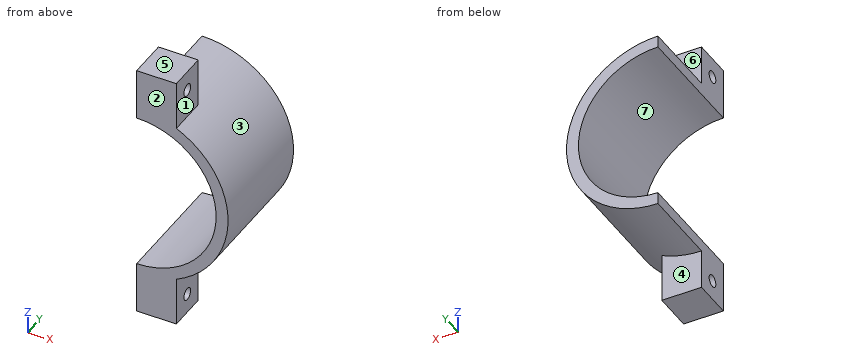
```python
from build123d import *

# Parameters (mm, degrees)
TUBE_DEPTH         = 30
TERMINALS_DEPTH    = 10
CUT_EXTRUDE1_REACH = 25
SKETCH3_R          = 1.524


with BuildPart() as part:
    # Sketch1 → Tube (new body)
    with BuildSketch(Plane(origin=(0, 0, 0), x_dir=(1, 0, 0), z_dir=(0, 1, 0))):
        with BuildLine():
            Line((0, 23), (0, 20))
            ThreePointArc((0, 20), (20, 0), (0, -20))
            Line((0, -20), (0, -23))
            ThreePointArc((0, -23), (23, 0), (0, 23))
        make_face()
    extrude(amount=TUBE_DEPTH)

    # Sketch2 → Terminals (add)
    with BuildSketch(Plane(origin=(0, 0, 0), x_dir=(-1, 0, 0), z_dir=(0, -1, 0))):
        with BuildLine():
            Line((0, -23), (0, -33))
            Line((0, -33), (-10, -33))
            Line((-10, -33), (-10, -20.712315177))
            ThreePointArc((-10, -20.712315177), (-5.129169081, -22.420785547), (0, -23))
        make_face()
        with BuildLine():
            Line((0, 23), (0, 33))
            Line((0, 33), (-10, 33))
            Line((-10, 33), (-10, 20.712315177))
            ThreePointArc((-10, 20.712315177), (-5.129169081, 22.420785547), (0, 23))
        make_face()
    extrude(amount=-TERMINALS_DEPTH)

    # Sketch3 → Cut-Extrude1 (cut, up to next)
    with BuildSketch(Plane.ZY, mode=Mode.PRIVATE) as cut_extrude1_sk1:
        with Locations((-28, 5)):
            Circle(SKETCH3_R)
    cut_extrude1_tool1 = extrude(cut_extrude1_sk1.sketch, amount=-CUT_EXTRUDE1_REACH, mode=Mode.PRIVATE) & part.part
    add(cut_extrude1_tool1.solids().sort_by_distance((0, 5, -28))[0], mode=Mode.SUBTRACT)
    # Sketch3 → Cut-Extrude1 (cut, up to next)
    with BuildSketch(Plane.ZY, mode=Mode.PRIVATE) as cut_extrude1_sk2:
        with Locations((28, 5)):
            Circle(SKETCH3_R)
    cut_extrude1_tool2 = extrude(cut_extrude1_sk2.sketch, amount=-CUT_EXTRUDE1_REACH, mode=Mode.PRIVATE) & part.part
    add(cut_extrude1_tool2.solids().sort_by_distance((0, 5, 28))[0], mode=Mode.SUBTRACT)


solid = part.part
```
Geometry: final body of the model. Coordinates: model frame, mm. Face numbers are marked on the shaded views. A direction names the side the tool comes from. Round coordinates to 2 decimals unless told otherwise and drop trailing zeros. Order: outer loops, then holes, each group sorted by start corner. A loop starts at its lowest first (then second) coordinate and runs counter-clockwise, first axis right, second up. Notation, with made-up numbers: M 11.5,73 L 58.5,73 A17 cw 58.5,84 Z; hole C 21,50.5 d2. An arc over 180 degrees is marked long. One line per item, written item: value.
(1) Line query: probe 1 along Y at (x, z) = (2, -28); probe 2 along Z at (x, y) = (15, 17.75); probe 3 along Z at (x, y) = (18.25, 21.25). Output: solid intervals per line, ascending. Write a range as [from, to].
Result sheet:
probe 1: [0, 3.48], [6.52, 10]
probe 2: [-17.44, -13.23], [13.23, 17.44]
probe 3: [-14, -8.18], [8.18, 14]
(2) Cut plane C-C (x = 14.5). Return the cut outline in (y, z).
Result sheet:
outline: M 0,-17.85 L 30,-17.85 L 30,-13.77 L 0,-13.77 Z; M 0,13.77 L 30,13.77 L 30,17.85 L 0,17.85 Z
(3) Pull-direction query (Z, two-part tool) for the marked faces 5, 6 and 7; classes: pulls with the +Z half, pulls with the -Z half, needs draft (parallel to the pull), parting line crosses it, or undercut.
Result sheet:
face 5: pulls with the +Z half
face 6: needs draft
face 7: undercut
(4) Cut plane A-A (x = 7.75). Return the cut outline in (y, z), and give its area (3 significant figures).
Result sheet:
outline: M 0,-33 L 10,-33 L 10,-21.65 L 30,-21.65 L 30,-18.44 L 0,-18.44 Z; M 0,18.44 L 30,18.44 L 30,21.65 L 10,21.65 L 10,33 L 0,33 Z; hole C 5,-28 d3.05; hole C 5,28 d3.05
area: 405 mm2
(5) Cut plane B-B (z = 28). Return the cut outline in (x, y).
Result sheet:
outline: M 0,0 L 10,0 L 10,3.48 L 0,3.48 Z; M 0,6.52 L 10,6.52 L 10,10 L 0,10 Z
(6) Reachability of the marked faces 1, 2, 3 and 4 from +Z, -Z, +X, -X, +Y, -Y: full face, straight path, thin tool, end or side. Return the list, or none.
Result sheet:
face 1: +Z, +X, +Y, -Y
face 2: +Z, -Z, +X, -X, -Y
face 3: +X, +Y
face 4: -Z, +X, +Y
(7) Pin query (flat end, axial travel): P1, Ø11, axis at x = 7, z = -28, coming from the +Y side; P2, Ø1, axis at y = 18.5, z = -13.5, coming from the +X side; P3, Ø12, axis at x = 16.5, z = 15.5, coming from the -Y side; P4, Ø3, axis at y = 6, z = 3, coming from the +X side. Return the tip coordinate at first contact, or that it passes through.
Result sheet:
P1: y = 10
P2: x = 18.97
P3: y = 0
P4: x = 22.95
(8) Cut plane D-D (x = 3.75). Return the cut outline in (y, z).
Result sheet:
outline: M 0,-33 L 10,-33 L 10,-22.69 L 30,-22.69 L 30,-19.65 L 0,-19.65 Z; M 0,19.65 L 30,19.65 L 30,22.69 L 10,22.69 L 10,33 L 0,33 Z; hole C 5,-28 d3.05; hole C 5,28 d3.05
